Build history of the part. All positions in model axes, mm. Face numbers are marked on the shaded views. Give positions to 0.01 mm unless a question says otherwise; leave off trailing zeros. Loops run counter-clockwise (first coordinate to the right, second up) from the corner with the lowest first, then second, coordinate; pieces in that order, holes last.
1) Band-saw the part on B-B on x = 10.5. List the corners of the cut face in (y, z).
2) Band-saw the part on A-A on z = 0. List the corners of the cut face in (x, y).
3) Wall check: line 1 (Z direction, x = 12, y = 0); line 2 (Z direction, x = 17, y = -13.5); line 3 (Y direction, x = 23.5, z = -13). Give the ranges that are in metal, low to high.
4) Band-saw the part on C-C on x = 27. List the corners of the cut face in (y, z), then the cut area to 3 significant figures.
5) Flat gauge pins, fed straight in: P1, Ø12, axis at x = 4.5, y = -6, coming from the +Z side; P2, Ø3, axis at x = 11, y = -3.5, coming from the -Z side; P3, Ø6, axis at x = 27, z = 24, coming from the +Y side. Where does each tip first touch, or does it go through?
6) Two-plate mould, pull along Y, no slides. Class the marked faces 1, 2, 3 and 4: +Y half, -Y half, draft (parallel to the pull), parting line (faces both ways), or undercut.
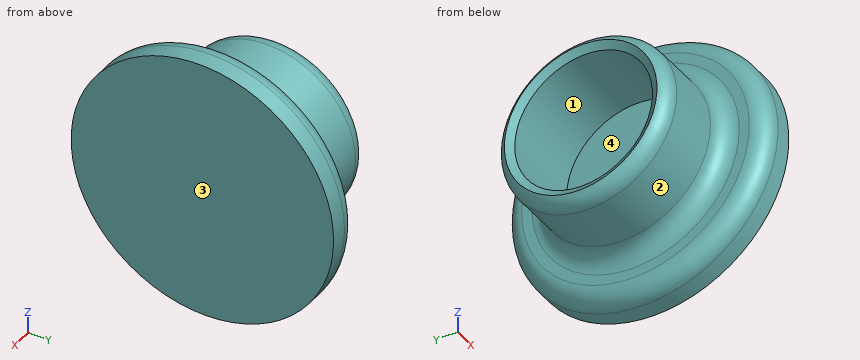
```python
from build123d import *

# Parameters (mm, degrees)
F0_R     = 25
F0_R_2   = 20
F1_DEPTH = 25.4
F2_R     = 38.1
F2_R_2   = 25
F2_R_3   = 20
F3_DEPTH = 10


# Not quite as in the source:
# - a fillet or chamfer that OpenCascade refuses, or shapes differently, is made with other operations: its cross-section is extruded or revolved along the edge and cut away or added


with BuildPart() as f1:
    # F0 (on Right) → F1 (new body)
    with BuildSketch(Plane.YZ):
        Circle(F0_R)
        Circle(F0_R_2, mode=Mode.SUBTRACT)
    extrude(amount=F1_DEPTH)

    # F2 (on face) → F3 (join)
    with BuildSketch(Plane.YZ.offset(25.4)):
        Circle(F2_R)
        Circle(F2_R_2, mode=Mode.SUBTRACT)
        Circle(F2_R_2)
        Circle(F2_R_3, mode=Mode.SUBTRACT)
        Circle(F2_R_3)
    extrude(amount=F3_DEPTH)

    # F4: fillet of radius 5.08 on 4 edges, made by hand

    # F4_s1 → F4_t2 (revolve)
    with BuildSketch(Plane.XY):
        with BuildLine():
            ThreePointArc((25.4, 30.08), (23.9121024484, 26.4878975516), (20.32, 25))
            Line((20.32, 25), (25.4, 25))
            Line((25.4, 25), (25.4, 30.08))
        make_face()
    revolve(axis=Axis((25.4, 0, 0), (1, 0, 0)))

    # F4_s3 → F4_t4 (revolve, cut)
    with BuildSketch(Plane.XY):
        with BuildLine():
            ThreePointArc((5.08, 25), (1.4878975516, 23.5121024484), (0, 19.92))
            Line((0, 19.92), (0, 25))
            Line((0, 25), (5.08, 25))
        make_face()
    revolve(axis=Axis((0, 0, 0), (1, 0, 0)), mode=Mode.SUBTRACT)

    # F4_s5 → F4_t6 (revolve, cut)
    with BuildSketch(Plane.XY):
        with BuildLine():
            ThreePointArc((30.48, 38.1), (26.8878975516, 36.6121024484), (25.4, 33.02))
            Line((25.4, 33.02), (25.4, 38.1))
            Line((25.4, 38.1), (30.48, 38.1))
        make_face()
    revolve(axis=Axis((25.4, 0, 0), (1, 0, 0)), mode=Mode.SUBTRACT)

    # F5: chamfer of 1.524 on 1 edges, made by hand

    # F5_s1 → F5_t2 (revolve, cut)
    with BuildSketch(Plane.XY):
        with BuildLine():
            Line((0.4894859208, 22.2141433772), (1.9000393506, 19.9482483046))
            Line((1.9000393506, 19.9482483046), (1.9000393506, 19.9177683046))
            ThreePointArc((1.9000393506, 19.9177683046), (0.9503346555, 19.96952), (0.0006299603, 19.96952))
            Line((0.0006299603, 19.96952), (-0.0298462599, 20.00048))
            ThreePointArc((-0.0298462599, 20.00048), (0.1169178679, 21.1385325522), (0.4621361335, 22.2275977273))
            Line((0.4621361335, 22.2275977273), (0.4894859208, 22.2141433772))
        make_face()
    revolve(axis=Axis((0.0006299603, 0, 0), (-1, 0, 0)), mode=Mode.SUBTRACT)


solid = f1.part
```
Findings below:
1. outline: circle Ø50 at (0, 0); hole circle Ø40 at (0, 0)
2. outline: (0.52, -22.16) arc R5.08 ccw to (5.08, -25) - (20.32, -25) arc R5.08 cw to (25.4, -30.08) - (25.4, -33.02) arc R5.08 ccw to (30.48, -38.1) - (35.4, -38.1) - (35.4, 38.1) - (30.48, 38.1) arc R5.08 ccw to (25.4, 33.02) - (25.4, 30.08) arc R5.08 cw to (20.32, 25) - (5.08, 25) arc R5.08 ccw to (0.52, 22.16) - (1.87, 20) - (25.4, 20) - (25.4, -20) - (1.87, -20) - close
3. line 1: z = -25 to -20, 20 to 25
3. line 2: z = -21.04 to -14.76, 14.76 to 21.04
3. line 3: y = -22.65 to -15.2, 15.2 to 22.65
4. outline: circle Ø73.44 at (0, 0)
4. area: 4,240 mm2
5. P1: stops at z = 25
5. P2: stops at z = -24.92
5. P3: stops at y = 31.04
6. face 1: undercut
6. face 2: parting line
6. face 3: draft
6. face 4: undercut
